The model under review builds one solid part; all positions refer to its coordinate system, in mm. Give positions to 0.01 mm unless a question says otherwise; leave off trailing zeros. Order: outer loops, then holes, each group sorted by start corner. A loop starts at its lowest first (then second) coordinate and runs counter-clockwise, first axis right, second up. Notation, with made-up numbers: (50.5, 81.25) - (59.5, 81.25) arc R8 ccw to (59.5, 89.25) - close; hole circle Ø4 at (74.25, 41). An arc over 180 degrees is marked (long way). Put each result on its own line as item: value.
```python
from build123d import *

# Parameters (mm, degrees)
SKETCH1_W           = 23
SKETCH1_H           = 23
BOSS_EXTRUDE1_DEPTH = 23
SKETCH2_R           = 5
CUT_EXTRUDE1_DEPTH  = 23
CUT_EXTRUDE2_DEPTH  = 23
CHAMFER1_SIZE       = 1


with BuildPart() as part:
    # Sketch1 → Boss-Extrude1 (new body)
    with BuildSketch(Plane.XY):
        Rectangle(SKETCH1_W, SKETCH1_H)
    extrude(amount=BOSS_EXTRUDE1_DEPTH)

    # Sketch2 → Cut-Extrude1 (cut)
    with BuildSketch(Plane.XY.offset(23)):
        Circle(SKETCH2_R)
    extrude(amount=-CUT_EXTRUDE1_DEPTH, mode=Mode.SUBTRACT)

    # Sketch3 → Cut-Extrude2 (cut)
    with BuildSketch(Plane(origin=(0, 11.5, 0), x_dir=(1, 0, 0), z_dir=(0, 1, 0))):
        with BuildLine():
            ThreePointArc((5, -11.5), (3.535533906, -7.964466094), (0, -6.5))
            Line((0, -6.5), (0, -16.5))
            ThreePointArc((0, -16.5), (3.535533906, -15.035533906), (5, -11.5))
        make_face()
        with BuildLine():
            Line((0, -16.5), (0, -6.5))
            ThreePointArc((0, -6.5), (-5, -11.5), (0, -16.5))
        make_face()
    extrude(amount=-CUT_EXTRUDE2_DEPTH, mode=Mode.SUBTRACT)

    # Chamfer1
    chamfer1_edges = [part.edges().sort_by_distance(p)[0] for p in [
        (-11.5, 0, 23),
        (0, -11.5, 23),
        (11.5, 0, 23),
        (0, -11.5, 0),
        (-11.5, 0, 0),
        (0, 11.5, 0),
        (11.5, 0, 0),
        (0, 11.5, 23),
        (11.5, -11.5, 11.5),
        (-11.5, -11.5, 11.5),
        (-11.5, 11.5, 11.5),
        (11.5, 11.5, 11.5),
    ]]
    chamfer(chamfer1_edges, length=CHAMFER1_SIZE)


solid = part.part
```
(1) The part is to be moulded in two halves that separate along X. For faces 1 (the cylindrical face through (-4, 3, 5)), 2 (the flat face through (-0.1, -11, 0.5)), 3 (the flat face through (-10.9, -10.8, 0.7)), say which applies: pulls with the +X half, pulls with the -X half, needs draft (parallel to the pull), parting line crosses it, or undercut.
The answers:
face 1: undercut
face 2: needs draft
face 3: pulls with the -X half
(2) Take a section at A-A, the plane z = 19.25. Write out the cut boundary in (x, y).
The answers:
outline: (-11.5, -10.5) - (-10.5, -11.5) - (10.5, -11.5) - (11.5, -10.5) - (11.5, 10.5) - (10.5, 11.5) - (-10.5, 11.5) - (-11.5, 10.5) - close; hole circle Ø10 at (0, 0)
(3) Wall thickness on L1, parallel to X at y = -4, z = 11.5; L2, parallel to X at y = -3.5, z = 3: over which ranges is each line inside the solid? List them lowest first.
The answers:
L1: -11.5 to -5, 5 to 11.5
L2: -11.5 to -3.57, 3.57 to 11.5
(4) Take a section at B-B, the plane x = 4. Write out the cut boundary in (y, z), then the cut area to 3 significant figures.
The answers:
outline: (-11.5, 1) - (-10.5, 0) - (-3, 0) - (-3, 8.5) - (-11.5, 8.5) - close; (-11.5, 14.5) - (-3, 14.5) - (-3, 23) - (-10.5, 23) - (-11.5, 22) - close; (3, 0) - (10.5, 0) - (11.5, 1) - (11.5, 8.5) - (3, 8.5) - close; (3, 14.5) - (11.5, 14.5) - (11.5, 22) - (10.5, 23) - (3, 23) - close
area: 287 mm^2
(5) Take a section at C-C, the plane y = 5.75. Write out the cut boundary in (x, z), then the cut area to 3 significant figures.
The answers:
outline: (-11.5, 1) - (-10.5, 0) - (10.5, 0) - (11.5, 1) - (11.5, 22) - (10.5, 23) - (-10.5, 23) - (-11.5, 22) - close; hole circle Ø10 at (0, 11.5)
area: 448 mm^2
